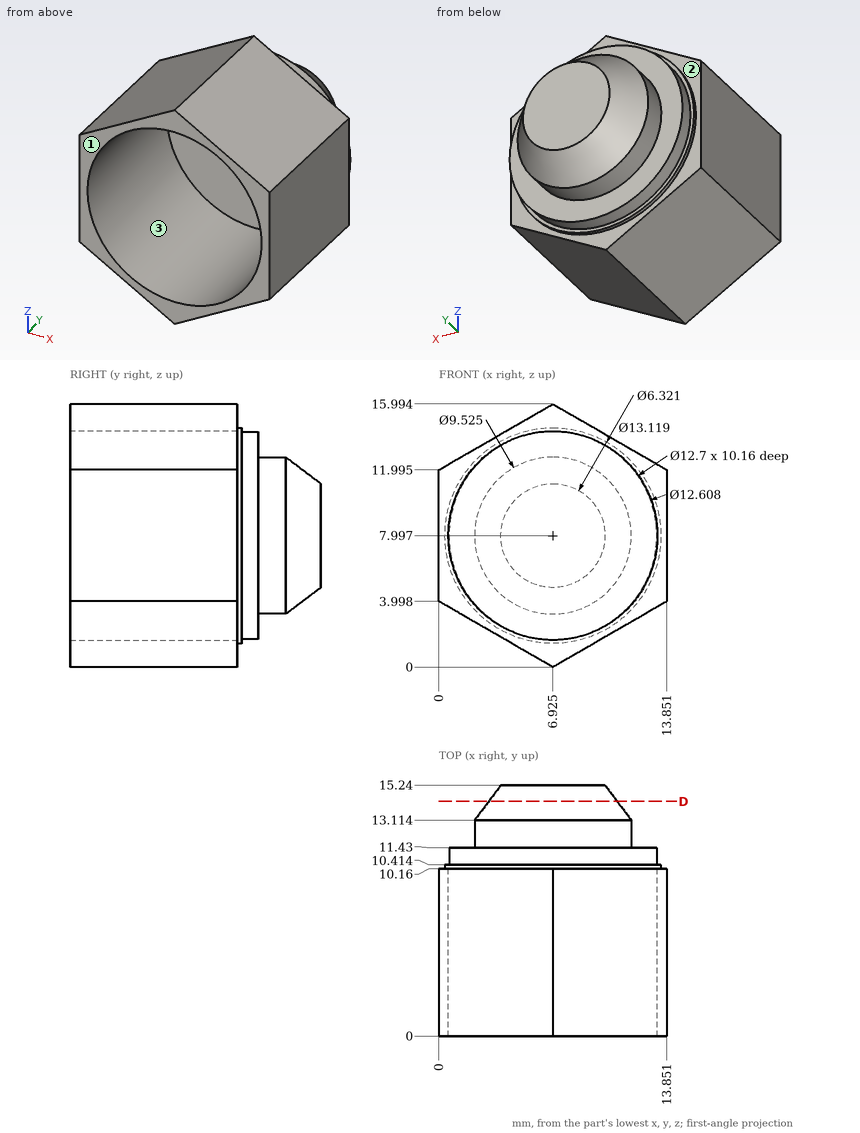
Answer from the drawing. Dimensions are ordinates in mm from the lowest x, y and z of the part. A direction names the side the tool comes from. Coordinates: 2 decimals unless noted, no trailing zeros. Order: outer loops, then holes, each group sorted by start corner. A loop starts at its lowest first (then second) coordinate and runs counter-clockwise, first axis right, second up. Notation, with made-up numbers: (28, 8) - (70, 8) arc R10 cw to (70, 15) - close; hole circle Ø7 at (-2, 46). An arc over 180 degrees is marked (long way). Answer as a JSON object with one key per item and string values. Group by question number.
Item 1: Flat-ended cylindrical pins translate along their axes: P1, Ø2, axis at x = 11, z = 1.5, coming from the +Y side; P2, Ø6.5, axis at x = 4, z = 8.5, coming from the -Y side; P3, Ø1, axis at x = 9.5, y = 8, coming from the -Z side. Find the tip coordinate at first contact, or state that the pin passes through.
Item 2: A tool of negligible diameter and unlimited length cuts with its end or side. For the marked faces 1, 2 and 3, from which of +Z, -Z, +X, -X, +Y, -Y can it reach the whole face along a straight path? Write none if from no direction.
Item 3: Section D-D (y = 14.25) is taken. Give the vertices of the cut face in (x, z) (1 decimal).
Item 4: Consider probe 1 along Y at (x, z) = (6.5, 7.25); probe 2 along X at (y, z) = (8.75, 8.75); probe 3 along X at (y, z) = (4.5, 6). Determine where each line is inside the solid, lowest interval first. Write a range as from..to.
Results are:
{
 "1": {"P1": "stops at y = 10.16", "P2": "stops at y = 10.16", "P3": "stops at z = 1.2"},
 "2": {"face 1": "+Z, -Z, +X, -X, -Y", "face 2": "+Y", "face 3": "-Y"},
 "3": {"outline": "circle Ø7.8 at (6.9, 8)"},
 "4": {"probe 1": "y = 10.16..15.24", "probe 2": "x = 0..0.62, 13.23..13.85", "probe 3": "x = 0..0.9, 12.95..13.85"}
}
